The listing builds one solid part. Answer for the finished solid, in the listing's coordinates (mm). Face numbers are marked on the shaded views. A direction names the side the tool comes from. Give positions to 0.01 mm unless a question says otherwise; leave off trailing zeros. Order: outer loops, then holes, each group sorted by start corner. A loop starts at its lowest first (then second) coordinate and runs counter-clockwise, first axis right, second up. Notation, with made-up numbers: (85, 50.25) - (137, 50.25) arc R23 cw to (137, 77.25) - close; hole circle Ø11 at (5, 49). An arc over 180 degrees is marked (long way). Answer in a Markdown table with one row per item.
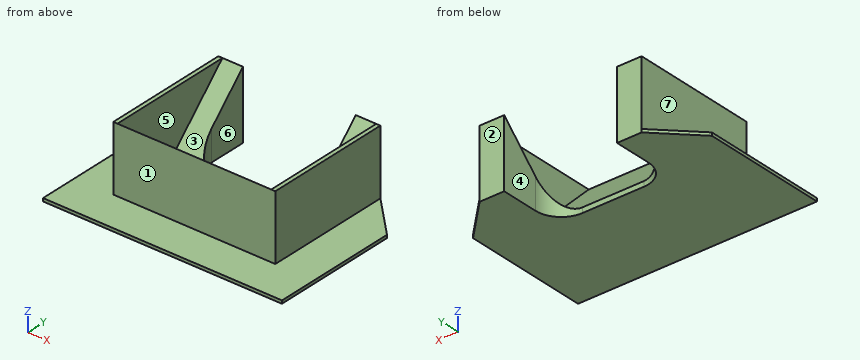
from build123d import *

# Parameters (mm, degrees)
BOSS_EXTRUDE1_DEPTH = 60
SKETCH2_W           = 44
SKETCH2_H           = 24.748737342
CUT_EXTRUDE1_DEPTH  = 27.748737342
FILLET1_R           = 10
SKETCH5_W           = 26.748737342
SKETCH5_H           = 49.497474684
BOSS_EXTRUDE3_DEPTH = 1.6
BOSS_EXTRUDE4_DEPTH = 1.2


with BuildPart() as part:
    # Sketch1 → Boss-Extrude1 (new body)
    with BuildSketch(Plane(origin=(0, 0, 0), x_dir=(0, 0, -1), z_dir=(1, 0, 0))):
        Polygon((-24.748737342, 24.748737342), (0, 0), (-24.748737342, -24.748737342), (2, -24.748737342), (2, 24.748737342), align=None)
    extrude(amount=BOSS_EXTRUDE1_DEPTH)

    # Sketch2 → Cut-Extrude1 (cut, through all)
    with BuildSketch(Plane(origin=(0, 0, -2), x_dir=(-1, 0, 0), z_dir=(0, 0, -1))):
        with Locations((-30, 12.374368671)):
            Rectangle(SKETCH2_W, SKETCH2_H)
    extrude(amount=-CUT_EXTRUDE1_DEPTH, mode=Mode.SUBTRACT)

    # Fillet1
    fillet1_edges = [part.edges().sort_by_distance(p)[0] for p in [
        (8, 0, -1),
        (52, 0, -1),
    ]]
    fillet(fillet1_edges, radius=FILLET1_R)

    # Sketch5 → Boss-Extrude3 (add)
    with BuildSketch(Plane.ZY):
        with Locations((11.374368671, 0)):
            Rectangle(SKETCH5_W, SKETCH5_H)
    boss_extrude3 = extrude(amount=BOSS_EXTRUDE3_DEPTH)

    # Mirror1: Boss-Extrude3 across plane
    add(boss_extrude3.mirror(Plane.ZY.offset(-30)))

    # Sketch6 → Boss-Extrude4 (add)
    with BuildSketch(Plane(origin=(0, 0, -2), x_dir=(-1, 0, 0), z_dir=(0, 0, -1))):
        Polygon((1.6, 24.748737342), (16.6, 9.748737342), (16.6, -39.748737342), (-76.6, -39.748737342), (-76.6, 9.748737342), (-61.6, 24.748737342), (-61.6, -24.748737342), (1.6, -24.748737342), align=None)
    extrude(amount=-BOSS_EXTRUDE4_DEPTH)


solid = part.part
Item 1: Determine the mould class of the marked faces 1, 2, 3 and 4 for opening direction Y: pulls with the +Y half, pulls with the -Y half, needs draft (parallel to the pull), parting line crosses it, or undercut.
Answer block:
| item | result |
|---|---|
| face 1 | pulls with the -Y half |
| face 2 | pulls with the +Y half |
| face 3 | undercut |
| face 4 | needs draft |
Item 2: Find section D-D on y = -19. Write down the section's boundary in (x, z).
Answer block:
| item | result |
|---|---|
| outline | (-16.6, -2) - (76.6, -2) - (76.6, -0.8) - (61.6, -0.8) - (61.6, 24.75) - (60, 24.75) - (60, 19) - (0, 19) - (0, 24.75) - (-1.6, 24.75) - (-1.6, -0.8) - (-16.6, -0.8) - close |
Item 3: Find section A-A on y = 4. Write down the section's boundary in (x, z), then the cut area to 3 significant figures.
Answer block:
| item | result |
|---|---|
| outline | (-16.6, -2) - (10, -2) - (10, 4) - (0, 4) - (0, 24.75) - (-1.6, 24.75) - (-1.6, -0.8) - (-16.6, -0.8) - close; (50, -2) - (76.6, -2) - (76.6, -0.8) - (61.6, -0.8) - (61.6, 24.75) - (60, 24.75) - (60, 4) - (50, 4) - close |
| area | 242 mm² |
Item 4: Consider line 1 (X direction, y = -12.5, z = 20.5); line 2 (X direction, y = 20, z = 16); line 3 (Z direction, x = 72, y = -32). Determine where each line is inside the solid, lowest interval first.
Answer block:
| item | result |
|---|---|
| line 1 | -1.6 to 0, 60 to 61.6 |
| line 2 | -1.6 to 8, 52 to 61.6 |
| line 3 | -2 to -0.8 |
Item 5: Find section B-B on z = 11.5. Write down the section's boundary in (x, y), then the cut area to 3 significant figures.
Answer block:
| item | result |
|---|---|
| outline | (-1.6, -24.75) - (61.6, -24.75) - (61.6, 24.75) - (52, 24.75) - (52, 11.5) - (60, 11.5) - (60, -11.5) - (0, -11.5) - (0, 11.5) - (8, 11.5) - (8, 24.75) - (-1.6, 24.75) - close |
| area | 1,170 mm² |
Item 6: Find section C-C on x = 56.5. Write down the section's boundary in (y, z), then the cut area to 3 significant figures.
Answer block:
| item | result |
|---|---|
| outline | (-39.75, -2) - (24.75, -2) - (24.75, 24.75) - (0, 0) - (-24.75, 24.75) - (-24.75, -0.8) - (-39.75, -0.8) - close |
| area | 729 mm² |
Item 7: Each of these flat-tipped pins is pushed along its axis until it touches: P1, Ø2, axis at x = 59, z = 7.5, coming from the -Y side; P2, Ø12, axis at y = 0.5, z = 19, coming from the +X side; P3, Ø1, axis at x = 45, z = 16.5, coming from the +Y side. Where does it stop, or does it pass through?
Answer block:
| item | result |
|---|---|
| P1 | y = -24.75 |
| P2 | x = 61.6 |
| P3 | y = -16 |
Item 8: Which of the six approach directions +Z, -Z, +X, -X, +Y, -Y give full straight-line access (tool end or side, diameter ignored) to the marked faces 5, 6 and 7?
Answer block:
| item | result |
|---|---|
| face 5 | +Z |
| face 6 | +Z, -Z, +Y |
| face 7 | +Z, -X, +Y, -Y |
